Here's how the part is built. I have some questions about the finished solid (model axes, mm). Give positions to 0.01 mm unless a question says otherwise; leave off trailing zeros. Answer in a Markdown table with one row per item. Add a question column.
Item 1: If we section it at A-A (z = 0): Give the number of separate pieces and of enclosed holes in the cut face, then the cut area to 3 significant figures.
Item 2: For P1, Ø1.8, axis at y = -32, z = 1, coming from the +X side; P2, Ø1.8, axis at y = -32, z = -1.5, coming from the -X side, each with a flat end and sliding along its axis, tell me the tip position at first contact or that it passes through.
Item 3: If I drill on line 1 (Y direction, x = 176, z = 2.5); line 2 (Z direction, x = 176, y = 274); line 3 (X direction, y = 244.5, z = -2), over which ranges is the centre line in solid material (lowest first)?
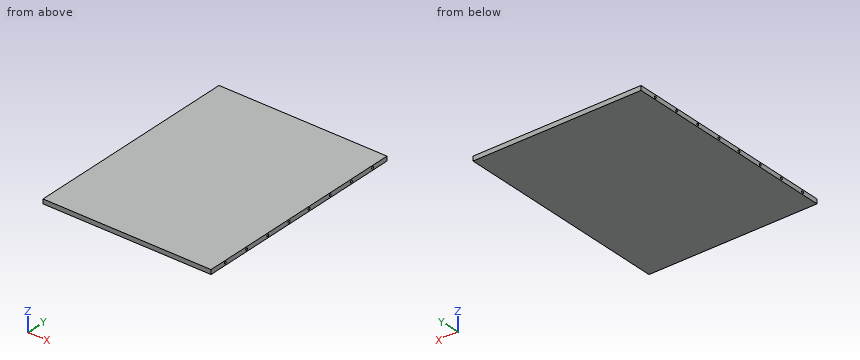
```python
from build123d import *

# Parameters (mm, degrees)
CROQUIS1_W              = 448
CROQUIS1_H              = 581
SALIENTE_EXTRUIR2_DEPTH = 6
CORTAR_EXTRUIR2_START   = 225
CROQUIS3_R              = 3
CORTAR_EXTRUIR2_DEPTH   = 27
CORTAR_EXTRUIR3_START   = 290
CROQUIS4_R              = 3
CORTAR_EXTRUIR3_DEPTH   = 27


with BuildPart() as part:
    # Croquis1 → Saliente-Extruir2 (new, symmetric)
    with BuildSketch(Plane.XY):
        Rectangle(CROQUIS1_W, CROQUIS1_H)
    extrude(amount=SALIENTE_EXTRUIR2_DEPTH, both=True)

    # Croquis3 → Cortar-Extruir2 (cut)
    with BuildSketch(Plane(origin=(0, 0, 0), x_dir=(0, 0, -1), z_dir=(1, 0, 0)).offset(CORTAR_EXTRUIR2_START)):
        with Locations((0, 243)):
            Circle(CROQUIS3_R)
        with Locations((0, 173)):
            Circle(CROQUIS3_R)
        with Locations((0, 103)):
            Circle(CROQUIS3_R)
        with Locations((0, 33)):
            Circle(CROQUIS3_R)
        with Locations(Location((0, -33, 0), (0, 0, 270))):
            Circle(CROQUIS3_R)
        with Locations(Location((0, -103, 0), (0, 0, 270))):
            Circle(CROQUIS3_R)
        with Locations(Location((0, -173, 0), (0, 0, 270))):
            Circle(CROQUIS3_R)
        with Locations(Location((0, -243, 0), (0, 0, 270))):
            Circle(CROQUIS3_R)
    cortar_extruir2 = extrude(amount=-CORTAR_EXTRUIR2_DEPTH, mode=Mode.SUBTRACT)

    # Simetría1: Cortar-Extruir2 across plane
    add(cortar_extruir2.mirror(Plane(origin=(0, 0, 0), x_dir=(0, 0, 1), z_dir=(1, 0, 0))), mode=Mode.SUBTRACT)

    # Croquis4 → Cortar-Extruir3 (cut)
    with BuildSketch(Plane(origin=(0, 0, 0), x_dir=(1, 0, 0), z_dir=(0, 1, 0)).offset(CORTAR_EXTRUIR3_START)):
        with Locations(Location((-176.5, 0, 0), (0, 0, 270))):
            Circle(CROQUIS4_R)
        with Locations(Location((-106.5, 0, 0), (0, 0, 270))):
            Circle(CROQUIS4_R)
        with Locations(Location((-36.5, 0, 0), (0, 0, 270))):
            Circle(CROQUIS4_R)
        with Locations(Location((36.5, 0, 0), (0, 0, 90))):
            Circle(CROQUIS4_R)
        with Locations(Location((106.5, 0, 0), (0, 0, 90))):
            Circle(CROQUIS4_R)
        with Locations(Location((176.5, 0, 0), (0, 0, 90))):
            Circle(CROQUIS4_R)
    cortar_extruir3 = extrude(amount=-CORTAR_EXTRUIR3_DEPTH, mode=Mode.SUBTRACT)

    # Simetría2: Cortar-Extruir3 across plane
    add(cortar_extruir3.mirror(Plane.ZX), mode=Mode.SUBTRACT)


solid = part.part
```
Recorded:
| question | item | result |
|---|---|---|
| 1 | separate pieces | 1 |
| 1 | enclosed holes | 12 |
| 1 | area | 256,000 mm^2 |
| 2 | P1 | stops at x = 198 |
| 2 | P2 | stops at x = -198 |
| 3 | line 1 | y = -290.5 to -290, -263 to 263, 290 to 290.5 |
| 3 | line 2 | z = -6 to -2.96, 2.96 to 6 |
| 3 | line 3 | x = -198 to 198 |
